Source: CAD feature listing. Evaluate the final solid. Frame: model axes, mm. Give positions to 0.01 mm unless a question says otherwise; leave off trailing zeros. Order: outer loops, then holes, each group sorted by start corner. A loop starts at its lowest first (then second) coordinate and runs counter-clockwise, first axis right, second up.
from build123d import *

# Parameters (mm, degrees)
EXTRUDE_1_DEPTH             = 40
HOLE_WIZARD_M3_1_AT_2_COUNT = 2
HOLE_WIZARD_M3_1_AT_2_PITCH = 17.556765078


with BuildPart() as part:
    # 草图1 → 凸台-拉伸1 (new body)
    with BuildSketch(Plane.XY):
        Polygon((8.237882641, -16.544998045), (-13.831826124, -34.234767829), (-30.256597299, -183.33281239), (6.654915402, -30.914593657), align=None)
    extrude(amount=EXTRUDE_1_DEPTH)

    # 草图5 → M3 螺纹孔1 (revolve, cut)
    with BuildSketch(Plane(origin=(-11.358047282, -41.00286285, 40), x_dir=(0, -1, 0), z_dir=(1, 0, 0))):
        Polygon((0, 0), (0, 8.251075774), (1.25, 7.5), (1.25, 0.275), (1.525, 0), align=None)
    hole_wizard_m3_1 = revolve(axis=Axis((-11.358047282, -41.00286285, 46.35), (0, 0, -1)), mode=Mode.SUBTRACT)

    # M3 螺纹孔1 at 2: M3 螺纹孔1 ×2
    with Locations(*[Vector(0.749142925, 0.662408392, 0) * (i * HOLE_WIZARD_M3_1_AT_2_PITCH) for i in range(1, HOLE_WIZARD_M3_1_AT_2_COUNT)]):
        add(hole_wizard_m3_1, mode=Mode.SUBTRACT)

    # 镜向1: M3 螺纹孔1 across plane
    add(hole_wizard_m3_1.mirror(Plane.XY.offset(20)), mode=Mode.SUBTRACT)

    # 镜向1 copy 1 sketch → 镜向1 copy 1 (revolve, cut)
    with BuildSketch(Plane(origin=(1.794479058, -29.373114321, 0), x_dir=(0, -1, 0), z_dir=(1, 0, 0))):
        Polygon((0, 0), (0, -8.251075774), (1.25, -7.5), (1.25, -0.275), (1.525, 0), align=None)
    revolve(axis=Axis((1.794479058, -29.373114321, -6.35), (0, 0, -1)), mode=Mode.SUBTRACT)


solid = part.part
1) Section query A-A on z = 37. Output: boundary loops of the cut face in (x, y) (3 decimals).
Checks:
outline: (-30.257, -183.333) - (6.655, -30.915) - (8.238, -16.545) - (-13.832, -34.235) - close; hole circle Ø2.5 at (-11.358, -41.003); hole circle Ø2.5 at (1.794, -29.373)
2) First-contact query: pin 1 Ø6 at (x, z) = (-11, 21) entering from +Y; pin 2 Ø2 at (x, y) = (1.79, -29.37) entering from -Z; pin 3 Ø4 at (x, z) = (-14, 15.5) entering from +Y; pin 4 Ø8 at (x, y) = (-14.5, -127) entering from -Z. Flat tips, straight axial feed; report the tip coordinate or a pass-through.
Checks:
pin 1: stops at y = -29.56
pin 2: stops at z = 7.65
pin 3: stops at y = -32.77
pin 4: stops at z = 0
3) Ray query, L1, parallel to X at y = -83, z = 6; L2, parallel to X at y = -70, z = 10. Return the intervals inside material, ascending.
Checks:
L1: x = -19.2 to -5.96
L2: x = -17.77 to -2.81
4) Section query C-C on y = -37.5. Output: boundary loops of the cut face in (x, z).
Checks:
outline: (-14.19, 0) - (5.06, 0) - (5.06, 40) - (-14.19, 40) - close
5) Section query B-B on x = -7.5. Output: boundary loops of the cut face in (y, z).
Checks:
outline: (-89.36, 0) - (-29.16, 0) - (-29.16, 40) - (-89.36, 40) - close
